Geometry: see drawing. Coordinates: mm, zero at the bounding-box minimum. Coordinates: 2 decimals unless noted, no trailing zeros. Write each loop counter-clockwise with the first axis right and the second up, starting at its lowest first coordinate (ties: lowest second). Pieces come first, ordered by that corner, then holes. Notation, with made-up numbers: (64.25, -40) - (119.25, -40) arc R11 cw to (119.25, -29) - close; hole circle Ø10 at (48, 79). An arc over 180 degrees is marked (long way). Use a Markdown table: item, result. Add a question column.
Q1. Pin query (flat end, axial travel): P1, Ø0.5, axis at y = 14, z = 11, coming from the +X side; P2, Ø0.5, axis at x = 32, z = 11, coming from the -Y side; P3, Ø0.5, axis at x = 32.5, z = 10.5, coming from the +Y side. Return the tip coordinate at first contact, or that it passes through.
Q2. Section query D-D (z = 8.25). Return the cut outline in (x, y), then the cut area to 3 significant figures.
Q3. Section query A-A (x = 36). Return the cut outline in (y, z) (1 decimal), then the cut area to 3 significant figures.
Q4. Section query C-C (z = 2.25). Return the cut outline in (x, y), then the cut area to 3 significant figures.
Q5. Material intervals for probe 1 along Z at (x, y) = (48, 45.5); probe 2 along X at (y, z) = (50.5, 8) (1 decimal); probe 3 along X at (y, z) = (12, 4.5), sorted ascending. Write a range as from..to.
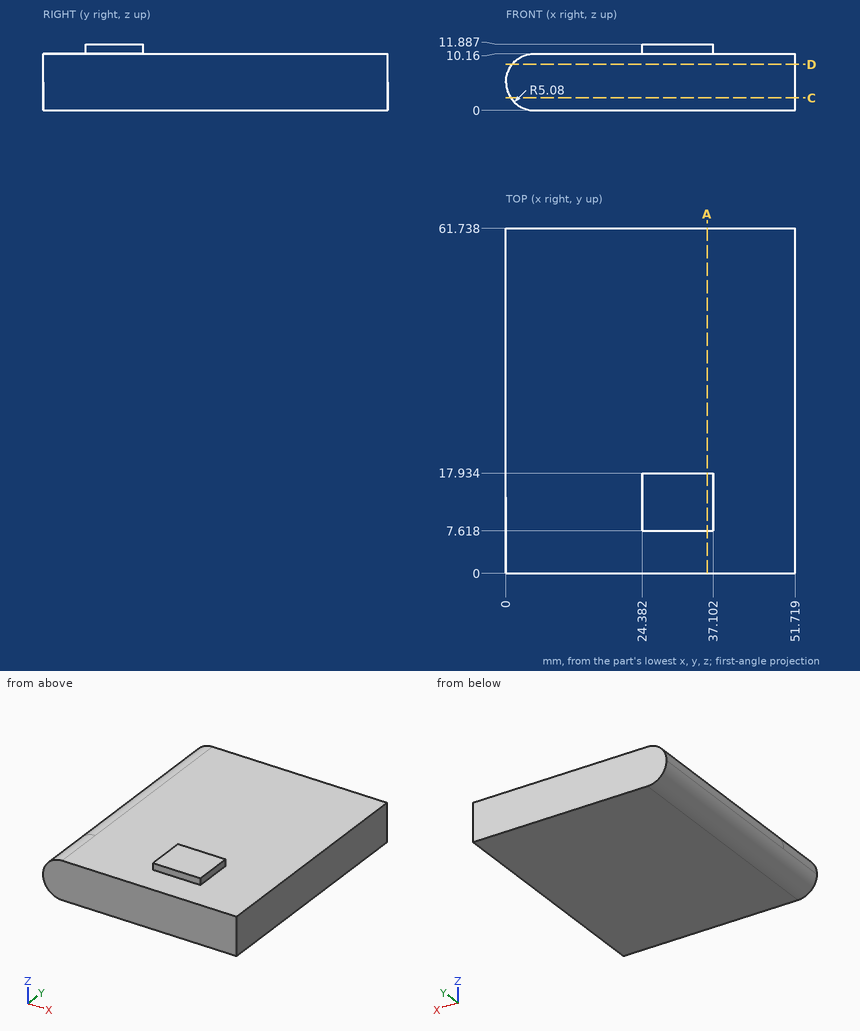
Values follow:
| question | item | result |
|---|---|---|
| 1 | P1 | x = 37.1 |
| 1 | P2 | y = 7.62 |
| 1 | P3 | y = 17.93 |
| 2 | outline | (1.11, 0) - (51.72, 0) - (51.72, 61.74) - (1.11, 61.74) - close |
| 2 | area | 3,120 mm2 |
| 3 | outline | (0, 0) - (61.7, 0) - (61.7, 10.2) - (17.9, 10.2) - (17.9, 11.9) - (7.6, 11.9) - (7.6, 10.2) - (0, 10.2) - close |
| 3 | area | 645 mm2 |
| 4 | outline | (0.86, 0) - (51.72, 0) - (51.72, 61.74) - (0.86, 61.74) - close |
| 4 | area | 3,140 mm2 |
| 5 | probe 1 | 0..10.16 |
| 5 | probe 2 | 0.9..51.7 |
| 5 | probe 3 | 0.03..51.72 |
